CAD build for the part. Positions are in the model's coordinates, mm. Face numbers are marked on the shaded views. A direction names the side the tool comes from. Round coordinates to 2 decimals unless told otherwise and drop trailing zeros. Loops run counter-clockwise (first coordinate to the right, second up) from the corner with the lowest first, then second, coordinate; pieces in that order, holes last.
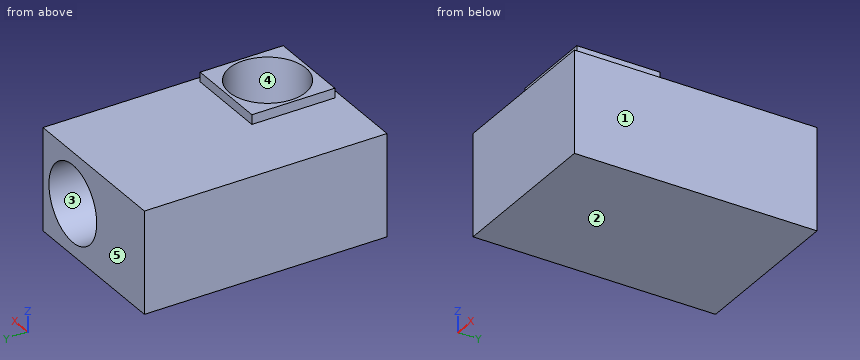
```python
from build123d import *

# Parameters (mm, degrees)
SKETCH1_W           = 6.375
SKETCH1_H           = 9.5
BOSS_EXTRUDE1_DEPTH = 4
SCALE1_SCALE        = 25.4
SKETCH3_W           = 82.55
SKETCH3_H           = 82.55
BOSS_EXTRUDE2_DEPTH = 9.525
SKETCH4_R           = 38.1
CUT_EXTRUDE1_DEPTH  = 101.6
SKETCH5_R           = 38.1
CUT_EXTRUDE2_DEPTH  = 101.6


with BuildPart() as part:
    # Sketch1 → Boss-Extrude1 (new body)
    with BuildSketch(Plane.XY):
        with Locations((-3.1875, 4.75)):
            Rectangle(SKETCH1_W, SKETCH1_H)
    extrude(amount=BOSS_EXTRUDE1_DEPTH)


with BuildPart() as part_1:
    # Scale1: scaled about (-3.1875, 4.75, 2)
    add(part.part.scale(SCALE1_SCALE).moved(Location((77.775, -115.9, -48.8))))

    # Sketch3 → Boss-Extrude2 (add)
    with BuildSketch(Plane.XY.offset(52.8)):
        with Locations((30.15, -68.275)):
            Rectangle(SKETCH3_W, SKETCH3_H)
    extrude(amount=BOSS_EXTRUDE2_DEPTH)

    # Sketch4 → Cut-Extrude1 (cut)
    with BuildSketch(Plane.XY.offset(62.325)):
        with Locations((30.15, -68.275)):
            Circle(SKETCH4_R)
    extrude(amount=-CUT_EXTRUDE1_DEPTH, mode=Mode.SUBTRACT)

    # Sketch5 → Cut-Extrude2 (cut)
    with BuildSketch(Plane(origin=(0, 125.4, 0), x_dir=(1, 0, 0), z_dir=(0, 1, 0))):
        with Locations((30.15, -2)):
            Circle(SKETCH5_R)
    extrude(amount=-CUT_EXTRUDE2_DEPTH, mode=Mode.SUBTRACT)


solid = part_1.part
```
Item 1: Cut at B-B, the plane z = 2. Give the cut face in (x, y) (3 decimals).
Answers follow:
outline: (-84.15, -115.9) - (77.775, -115.9) - (77.775, 125.4) - (68.25, 125.4) - (68.25, 23.8) - (-7.95, 23.8) - (-7.95, 125.4) - (-84.15, 125.4) - close; hole circle Ø76.2 at (30.15, -68.275)
Item 2: Cut at C-C, the plane y = 110.5. Give the cut face in (x, z) (3 decimals).
Answers follow:
outline: (-84.15, -48.8) - (77.775, -48.8) - (77.775, 52.8) - (-84.15, 52.8) - close; hole circle Ø76.2 at (30.15, 2)
Item 3: Cut at A-A, the plane x = 30.15. Give the cut face in (y, z) (3 decimals).
Answers follow:
outline: (-115.9, -48.8) - (125.4, -48.8) - (125.4, -36.1) - (23.8, -36.1) - (23.8, 40.1) - (125.4, 40.1) - (125.4, 52.8) - (-27, 52.8) - (-27, 62.325) - (-30.175, 62.325) - (-30.175, -39.275) - (-106.375, -39.275) - (-106.375, 62.325) - (-109.55, 62.325) - (-109.55, 52.8) - (-115.9, 52.8) - close
Item 4: Probe line 1 (X direction, y = 98, z = 2) (3 decimals); line 2 (Z direction, x = 30.15, y = 54.5); line 3 (Y direction, x = 30.15, z = 27) (3 decimals). List the from-to ranges inside material, lowest first.
Answers follow:
line 1: x = -84.15 to -7.95, 68.25 to 77.775
line 2: z = -48.8 to -36.1, 40.1 to 52.8
line 3: y = -115.9 to -106.375, -30.175 to 23.8
Item 5: 3-axis set-ups, long thin cutter, end or side, ignore diameter. For the marked faces 4 and 5: which of +Z, -Z, +X, -X, +Y, -Y reach the whole face in a straight line?
Answers follow:
face 4: +Z
face 5: +Z, -Z, +X, -X, +Y
Item 6: Two-plate mould, pull along Z, no slides. Class the marked faces 1, 2 and 3: released by +Z, released by -Z, zero draft, split by the parting line, or undercut.
Answers follow:
face 1: zero draft
face 2: released by -Z
face 3: undercut
Item 7: Flat gauge pins, fed straight in: P1, Ø5, axis at y = -85, z = 57, coming from the -X side (3 decimals); P2, Ø1, axis at x = -23, y = -23, coming from the +Z side; P3, Ø10.5, axis at x = 28.5, z = 59.5, coming from the -Y side. Where does each tip first touch, or does it go through?
Answers follow:
P1: stops at x = -11.125
P2: stops at z = 52.8
P3: stops at y = -109.55
Item 8: Cut at D-D, the plane y = -92. Give the cut face in (x, z) (3 decimals).
Answers follow:
outline: (-84.15, -48.8) - (77.775, -48.8) - (77.775, 52.8) - (71.425, 52.8) - (71.425, 62.325) - (59.962, 62.325) - (59.962, -39.275) - (0.338, -39.275) - (0.338, 62.325) - (-11.125, 62.325) - (-11.125, 52.8) - (-84.15, 52.8) - close
